```python
from build123d import *

# Parameters (mm, degrees)
EXTRUDE_1_DEPTH = 15.8
FILLET_1_R      = 3
M4X0_71_D       = 3.3
CHAMFER_1_SIZE  = 0.5
CHAMFER_1_SIZE2 = 1


with BuildPart() as part:
    # Эскиз1 → Бобышка-Вытянуть1 (new body)
    with BuildSketch(Plane(origin=(0, 0, 0), x_dir=(1, 0, 0), z_dir=(0, 1, 0))):
        Polygon((0, 0), (0, 5), (-13.886751346, 5), (-11, 0), align=None)
    extrude(amount=EXTRUDE_1_DEPTH)

    # Скругление1
    fillet_1_edges = [part.edges().sort_by_distance(p)[0] for p in [
        (0, 0, -2.5),
        (0, 15.8, -2.5),
    ]]
    fillet(fillet_1_edges, radius=FILLET_1_R)

    # Отверстие обработанное метчиком M4x0.71 (through all)
    with Locations(Plane.XY):
        with Locations((-5, 7.9)):
            Hole(M4X0_71_D / 2)

    # Фаска1
    chamfer_1_edges = [part.edges().sort_by_distance(p)[0] for p in [
        (-13.886751346, 7.9, -5),
    ]]
    chamfer_1_side = [part.faces().sort_by_distance(p)[0] for p in [
        (-7.140744189, 7.9, -5),
    ]]
    chamfer(chamfer_1_edges, length=CHAMFER_1_SIZE, length2=CHAMFER_1_SIZE2, reference=chamfer_1_side[0])


solid = part.part
```
Work out the finished part from the listing and answer in its coordinate system (mm). Coordinates: 2 decimals unless noted, no trailing zeros. Loops run counter-clockwise (first coordinate to the right, second up) from the corner with the lowest first, then second, coordinate; pieces in that order, holes last.
1) Consider probe 1 along Y at (x, z) = (-5, -3.35); probe 2 along Y at (x, z) = (-6.5, -1.45); probe 3 along X at (y, z) = (11.25, -0.65). Determine where each line is inside the solid, lowest interval first.
Results:
probe 1: y = 0 to 6.25, 9.55 to 15.8
probe 2: y = 0 to 7.21, 8.59 to 15.8
probe 3: x = -11.38 to 0
2) For a pull along X with two mould halves and no side action, classify faces 1 (the flat face through (-8, 8, -5)), 2 (the cylindrical face through (-0.86, 0.9, -2.54)), 3 (the cylindrical face through (-3.69, 6.9, -2.54)) as +X half, -X half, draft (parallel to the pull), parting line (faces both ways), or undercut.
Results:
face 1: draft
face 2: +X half
face 3: undercut
3) A flat-ended cylindrical pin translates along its axis: pin 1 (2 mm diameter, centred on x = -1.5, z = -3.5, fed in from -Y). Find the tip coordinate at first contact, or state that the pin passes through.
Results:
pin 1: stops at y = 0.04
4) Section B-B (x = -5) is taken. Give the vertices of the cut face in (y, z).
Results:
outline: (0, -5) - (6.25, -5) - (6.25, 0) - (0, 0) - close; (9.55, -5) - (15.8, -5) - (15.8, 0) - (9.55, 0) - close
5) Section D-D (y = 6) is taken. Give the vertices of the cut face in (x, z), plus the area to 3 significant figures.
Results:
outline: (-13.39, -5) - (0, -5) - (0, 0) - (-11, 0) - (-13.39, -4.13) - close
area: 62.0 mm2
6) Section C-C (z = -1.15) is taken. Give the vertices of the cut face in (x, y).
Results:
outline: (-11.66, 0) - (-3, 0) arc R3 ccw to (0, 3) - (0, 12.8) arc R3 ccw to (-3, 15.8) - (-11.66, 15.8) - close; hole circle Ø3.3 at (-5, 7.9)
7) Section A-A (y = 7.9) is taken. Give the vertices of the cut face in (x, z).
Results:
outline: (-13.39, -5) - (-6.65, -5) - (-6.65, 0) - (-11, 0) - (-13.39, -4.13) - close; (-3.35, -5) - (0, -5) - (0, 0) - (-3.35, 0) - close
